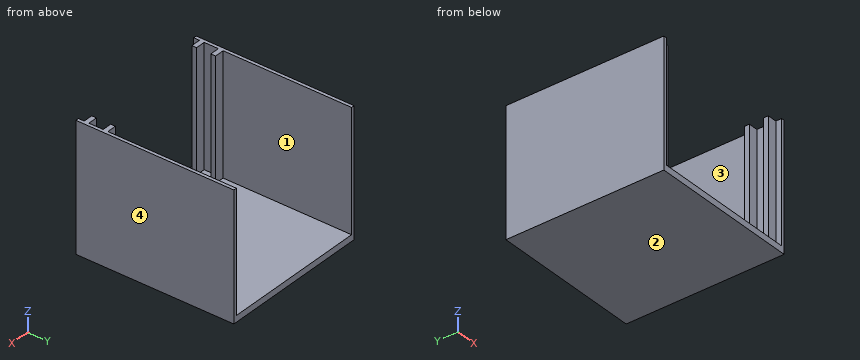
```python
from build123d import *

# Parameters (mm, degrees)
SKETCH1_W           = 48
SKETCH1_H           = 50
BOSS_EXTRUDE1_DEPTH = 40
CUT_EXTRUDE5_START  = 40
CUT_EXTRUDE5_DEPTH  = 38


with BuildPart() as part:
    # Sketch1 → Boss-Extrude1 (new body)
    with BuildSketch(Plane.XY):
        with Locations((0, 2.677885393)):
            Rectangle(SKETCH1_W, SKETCH1_H)
    extrude(amount=BOSS_EXTRUDE1_DEPTH)

    # Sketch4 → Cut-Extrude5 (cut)
    with BuildSketch(Plane.XY.offset(CUT_EXTRUDE5_START)):
        Polygon((-23, -19), (-23, -14.5), (-20, -14.5), (-20, -13), (-23, -13), (-23, 27.677885393), (23, 27.677885393), (23, -13), (20, -13), (20, -14.5), (23, -14.5), (23, -19), (20, -19), (20, -20.5), (23, -20.5), (23, -22.322114607), (-23, -22.322114607), (-23, -20.5), (-20, -20.5), (-20, -19), align=None)
    extrude(amount=-CUT_EXTRUDE5_DEPTH, mode=Mode.SUBTRACT)


solid = part.part
```
Design review of the part built by this model. Coordinates are the model's own, in mm. Face numbers are marked on the shaded views. Coordinates: 2 decimals unless noted, no trailing zeros. Loops run counter-clockwise (first coordinate to the right, second up) from the corner with the lowest first, then second, coordinate; pieces in that order, holes last. Notation, with made-up numbers: (17, -15) - (67, -15) arc R29 cw to (67, 20) - close; hole circle Ø6 at (30, -14). An arc over 180 degrees is marked (long way). Use CSV: the item, a comma, the result in double quotes. Start each with the question number.
1) Consider section B-B on y = -2. Write out the cut boundary in (x, z), then the cut area to 3 significant figures.
2) The part is to be moulded in two halves that separate along X. For the marked faces 1, 2, 3 and 4, say which applies: +X half, -X half, draft (parallel to the pull), parting line (faces both ways), or undercut.
3) Wall thickness on L1, parallel to X at y = 16, z = 25; L2, parallel to Z at x = 6.5, y = 21: over which ranges is each line inside the solid? List them lowest first. Write a range as from..to.
4) Consider section A-A on z = 13. Write out the cut boundary in (x, y), then the cut area to 3 significant figures.
5) For pin 1 Ø3.5 at (x, z) = (-22, 12.5) entering from -Y; pin 2 Ø1.5 at (x, z) = (21.5, 26) entering from -Y; pin 3 Ø3.5 at (x, z) = (-21, 30) entering from +Y, all flat-tipped, find the tip position at first contact; note any pin that passes through.
6) Consider section C-C on x = 7.5. Write out the cut boundary in (y, z).
Geometry says:
1,outline,"(-24, 0) - (24, 0) - (24, 40) - (23, 40) - (23, 2) - (-23, 2) - (-23, 40) - (-24, 40) - close"
1,area,"172 mm^2"
2,face 1,"undercut"
2,face 2,"draft"
2,face 3,"undercut"
2,face 4,"+X half"
3,L1,"-24..-23, 23..24"
3,L2,"0..2"
4,outline,"(-24, -22.32) - (-23, -22.32) - (-23, -20.5) - (-20, -20.5) - (-20, -19) - (-23, -19) - (-23, -14.5) - (-20, -14.5) - (-20, -13) - (-23, -13) - (-23, 27.68) - (-24, 27.68) - close; (20, -20.5) - (23, -20.5) - (23, -22.32) - (24, -22.32) - (24, 27.68) - (23, 27.68) - (23, -13) - (20, -13) - (20, -14.5) - (23, -14.5) - (23, -19) - (20, -19) - close"
4,area,"118 mm^2"
5,pin 1,"y = -22.32"
5,pin 2,"y = -20.5"
5,pin 3,"y = -13"
6,outline,"(-22.32, 0) - (27.68, 0) - (27.68, 2) - (-22.32, 2) - close"
